Geometry: final body of the model. Coordinates: model frame, mm. Coordinates: 2 decimals unless noted, no trailing zeros. Loops run counter-clockwise (first coordinate to the right, second up) from the corner with the lowest first, then second, coordinate; pieces in that order, holes last. Notation, with made-up numbers: (56, 12) -> (107, 12) arc R20 cw to (107, 19) -> close; hole circle Ø2 at (-11, 31.25). An arc over 180 degrees is marked (long way). One line per item, written item: value. Start each with the question number.
Autodesk Inventor part; units mm, degrees
ref_plane "YZ Plane" through (0, 0, 0) normal (1, 0, 0) x (0, 1, 0)
ref_plane "XZ Plane" through (0, 0, 0) normal (0, 1, 0) x (-1, 0, 0)
ref_plane "XY Plane" through (0, 0, 0) normal (0, 0, 1) x (1, 0, 0)
sketch "Sketch1" plane through (0, 0, 0) normal (0, 0, 1) x (1, 0, 0)
  line L0 (0, 0) -> (25.4, 0)
  line L1 (25.4, 0) -> (25.4, 258.7625)
  line L2 (25.4, 258.7625) -> (0, 258.7625)
  line L3 (0, 258.7625) -> (0, 0)
  line L4 (12.7, 0) -> (12.7, 207.9625) construction
  circle A0 centre (12.7, 207.9625) radius 9.525
  dimension "d0" = 25.4
  dimension "d1" = 258.7625
  dimension "d2" = 207.9625
  dimension "d3" = 19.05
extrude "Extrusion1" add sketch "Sketch1" along normal blind 3.175
properties part number "wall"
1. Draft query along X for faces 1 (the face through (11.46, 198.52, 1.57)), 2 (the face through (13, 131, 0)). Return one class per face: released by +X, released by -X, zero draft, split by the parting line, or undercut.
2. Section A-A on x = 12.7. Return the cut outline in (y, z) (1 decimal), plus the area to 3 significant figures.
3. Line query: L1, parallel to Y at x = 12.7, z = 0.7; L2, parallel to Y at x = 12, z = 0.85; L3, parallel to X at y = 216, z = 2.75. Output: solid intervals per line, ascending. Write a range as [from, to].
4. Section C-C on y = 201.5. Return the cut outline in (x, z) (3 decimals), plus the area to 3 significant figures.
Checks:
1. face 1: undercut
1. face 2: zero draft
2. outline: (0, 0) -> (198.4, 0) -> (198.4, 3.2) -> (0, 3.2) -> close; (217.5, 0) -> (258.8, 0) -> (258.8, 3.2) -> (217.5, 3.2) -> close
2. area: 761 mm²
3. L1: [0, 198.44], [217.49, 258.76]
3. L2: [0, 198.46], [217.46, 258.76]
3. L3: [0, 7.59], [17.81, 25.4]
4. outline: (0, 0) -> (5.703, 0) -> (5.703, 3.175) -> (0, 3.175) -> close; (19.697, 0) -> (25.4, 0) -> (25.4, 3.175) -> (19.697, 3.175) -> close
4. area: 36.2 mm²
